Could you check a few things on this model? Use its own coordinates, in mm. Face numbers are marked on the shaded views. A direction names the side the tool comes from. Give positions to 0.01 mm unless a question says otherwise; leave off trailing zeros. Loops run counter-clockwise (first coordinate to the right, second up) from the corner with the lowest first, then second, coordinate; pieces in that order, holes last. Notation, with made-up numbers: (87, 7) - (128, 7) arc R20 ccw to (128, 18) - close; hole circle Ø3 at (69, -30). An arc over 180 degrees is marked (long way). Write each question's results on one line, items separated by ' | '. Start each with the question number.
(1) Suppose I cut it at C-C (x = 34). Please give me the cut outline in (y, z).
(2) For pin 1 (2 mm diameter, centred on x = 33.5, z = 0.5, fed in from +Y); pin 2 (2 mm diameter, centred on y = 27, z = 1.5, fed in from -X); pin 3 (1 mm diameter, centred on x = 77, z = 1, fed in from -Y), each with a flat end and sliding along its axis, tell me the tip position at first contact or that it passes through.
(3) Suppose I cut it at B-B (y = 26.5). Please give me the cut outline in (x, z), and give its area (3 significant figures).
(4) Suppose I cut it at D-D (z = 13). Please give me the cut outline in (x, y).
(5) Suppose I cut it at A-A (z = 4.75). Please give me the cut outline in (x, y).
(6) On a 3-axis mill with a long thin cutter (end or side, diameter ignored), from which of +Z, -Z, +X, -X, +Y, -Y can I reach the whole of each face in a straight line? I mean the marked faces 1 and 2. Say none if no direction works.
(7) I need wall thicknesses on line 1 (X direction, y = 50.65, z = 13); line 2 (Y direction, x = 29, z = 16.25); line 3 (Z direction, x = 34.5, y = 9). Which ranges of each line are inside material? Lowest first, please.
from build123d import *

# Parameters (mm, degrees)
CYLINDER_R                = 2
CYLINDER_DEPTH            = 60
CYLINDER001_R             = 2
CYLINDER001_DEPTH         = 60
BOX003_W                  = 30
BOX003_H                  = 2
BOX003_DEPTH              = 20
FILLET002_R               = 1.9
FILLET004_R               = 3
BOX004_W                  = 30
BOX004_H                  = 2
BOX004_DEPTH              = 20
FILLET003_R               = 1.9
FILLET003_PLACEMENT_ANGLE = 180.1
FILLET005_R               = 3
BOX001_W                  = 40
BOX001_H                  = 30
BOX001_DEPTH              = 10
BOX002_W                  = 20
BOX002_H                  = 30
BOX002_DEPTH              = 10
BOX_W                     = 100
BOX_H                     = 50
BOX_DEPTH                 = 2
FILLET_R                  = 3
FILLET001_R               = 3
FILLET006_R               = 1.25


with BuildPart() as cylinder:
    # Cylinder → Cylinder (new body)
    with BuildSketch(Plane(origin=(7, -6, 13), x_dir=(1, 0, 0), z_dir=(0, 1, 0))):
        Circle(CYLINDER_R)
    extrude(amount=CYLINDER_DEPTH)


with BuildPart() as fusion002:
    # Cylinder001 → Cylinder001 (new body)
    with BuildSketch(Plane(origin=(23, -6, 13), x_dir=(1, 0, 0), z_dir=(0, 1, 0))):
        Circle(CYLINDER001_R)
    extrude(amount=CYLINDER001_DEPTH)

    # Fusion002: union Cylinder
    add(cylinder.part)


with BuildPart() as fillet004:
    # Box003 → Box003 (new body)
    with BuildSketch(Plane(origin=(0, -1, 2), x_dir=(1, 0, 0), z_dir=(0, 0, 1))):
        with Locations((15, 1)):
            Rectangle(BOX003_W, BOX003_H)
    extrude(amount=BOX003_DEPTH)

    # Fillet002
    fillet002_edges = [fillet004.edges().sort_by_distance(p)[0] for p in [
        (15, -1, 2),
    ]]
    fillet(fillet002_edges, radius=FILLET002_R)


with BuildPart() as fillet004_1:
    # Fillet002 placement: moved
    add(fillet004.part.moved(Location((0, -1, -2))))

    # Fillet004
    fillet004_edges = [fillet004_1.edges().sort_by_distance(p)[0] for p in [
        (0, -1, 20),
        (30, -1, 20),
    ]]
    fillet(fillet004_edges, radius=FILLET004_R)


with BuildPart() as cut001:
    # Box004 → Box004 (new body)
    with BuildSketch(Plane(origin=(0, -1, 2), x_dir=(1, 0, 0), z_dir=(0, 0, 1))):
        with Locations((15, 1)):
            Rectangle(BOX004_W, BOX004_H)
    extrude(amount=BOX004_DEPTH)

    # Fillet003
    fillet003_edges = [cut001.edges().sort_by_distance(p)[0] for p in [
        (15, -1, 2),
    ]]
    fillet(fillet003_edges, radius=FILLET003_R)


with BuildPart() as cut001_1:
    # Fillet003 placement: moved
    add(cut001.part.moved(Location((29.889927, 50.903819, -2))).rotate(Axis((29.889927, 50.903819, -2), (0, 0, 1)), FILLET003_PLACEMENT_ANGLE))

    # Fillet005
    fillet005_edges = [cut001_1.edges().sort_by_distance(p)[0] for p in [
        (29.889927, 50.903819, 20),
        (-0.110027, 50.851459, 20),
    ]]
    fillet(fillet005_edges, radius=FILLET005_R)

    # Fusion001: union Fillet004
    add(fillet004_1.part)

    # Cut001: cut Fusion002
    add(fusion002.part, mode=Mode.SUBTRACT)


with BuildPart() as cube001:
    # Box001 → Box001 (new body)
    with BuildSketch(Plane(origin=(10, 10, -2), x_dir=(1, 0, 0), z_dir=(0, 0, 1))):
        with Locations((20, 15)):
            Rectangle(BOX001_W, BOX001_H)
    extrude(amount=BOX001_DEPTH)


with BuildPart() as fusion:
    # Box002 → Box002 (new body)
    with BuildSketch(Plane(origin=(70, 10, -2), x_dir=(1, 0, 0), z_dir=(0, 0, 1))):
        with Locations((10, 15)):
            Rectangle(BOX002_W, BOX002_H)
    extrude(amount=BOX002_DEPTH)

    # Fusion: union Cube001
    add(cube001.part)


with BuildPart() as fillet006:
    # Box → Box (new body)
    with BuildSketch(Plane.XY):
        with Locations((50, 25)):
            Rectangle(BOX_W, BOX_H)
    extrude(amount=BOX_DEPTH)

    # Cut: cut Fusion
    add(fusion.part, mode=Mode.SUBTRACT)

    # Fillet
    fillet_edges = [fillet006.edges().sort_by_distance(p)[0] for p in [
        (50, 10, 1),
        (10, 10, 1),
        (50, 40, 1),
        (10, 40, 1),
        (90, 10, 1),
        (70, 10, 1),
        (90, 40, 1),
        (70, 40, 1),
    ]]
    fillet(fillet_edges, radius=FILLET_R)

    # Fillet001
    fillet001_edges = [fillet006.edges().sort_by_distance(p)[0] for p in [
        (100, 50, 1),
        (100, 0, 1),
    ]]
    fillet(fillet001_edges, radius=FILLET001_R)

    # Fusion003: union Cut001
    add(cut001_1.part)

    # Fillet006
    fillet006_edges = [fillet006.edges().sort_by_distance(p)[0] for p in [
        (14.945836, 49.877735, 2),
        (15, 0, 2),
    ]]
    fillet(fillet006_edges, radius=FILLET006_R)


solid = fillet006.part
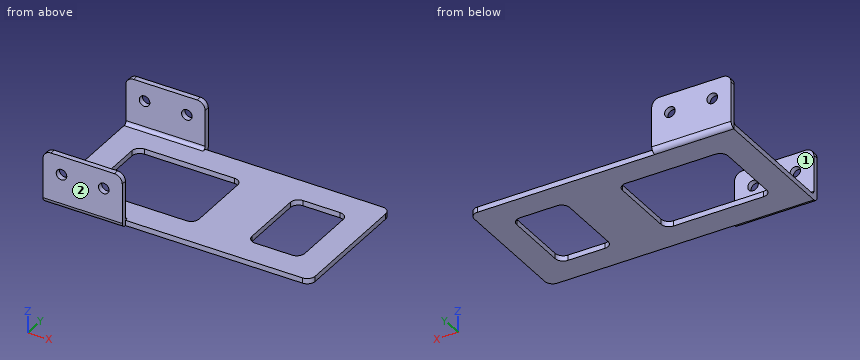
Output values:
1) outline: (0, 0) - (10, 0) - (10, 2) - (0, 2) - close; (40, 0) - (50, 0) - (50, 2) - (40, 2) - close
2) pin 1: y = 50 | pin 2: x = 0 | pin 3: y = 0
3) outline: (0, 0) - (10, 0) - (10, 2) - (0, 2) - close; (50, 0) - (70, 0) - (70, 2) - (50, 2) - close; (90, 0) - (100, 0) - (100, 2) - (90, 2) - close | area: 80.0 mm2
4) outline: (-0.11, 49.85) - (5, 49.86) - (5, 51.86) - (-0.11, 51.85) - close; (0, -2) - (5, -2) - (5, 0) - (0, 0) - close; (9, -2) - (21, -2) - (21, 0) - (9, 0) - close; (9, 49.87) - (21, 49.89) - (21, 51.89) - (9, 51.87) - close; (25, -2) - (30, -2) - (30, 0) - (25, 0) - close; (25, 49.9) - (29.89, 49.9) - (29.89, 51.9) - (25, 51.9) - close
5) outline: (-0.11, 49.85) - (29.89, 49.9) - (29.89, 51.9) - (-0.11, 51.85) - close; (0, -2) - (30, -2) - (30, 0) - (0, 0) - close
6) face 1: +Z, +X, -X | face 2: +Z, -Z, +X, -X, -Y
7) line 1: -0.11 to 5, 9 to 21, 25 to 29.89 | line 2: -2 to 0, 49.9 to 51.9 | line 3: 0 to 2
